from build123d import *

# Parameters (mm, degrees)
SKETCH2_R           = 3.175
SKETCH2_R_2         = 2
SKETCH2_R_3         = 1.905
SKETCH2_R_4         = 1.999999991
BOSS_EXTRUDE1_DEPTH = 5.588


with BuildPart() as part:
    # Sketch2 → Boss-Extrude1 (new body)
    with BuildSketch(Plane(origin=(0, 0, 0), x_dir=(1, 0, 0), z_dir=(0, 1, 0))):
        with BuildLine():
            Line((15.15555913, -28.018449791), (13.238676936, -27.713033224))
            ThreePointArc((13.238676936, -27.713033224), (11.241051513, -26.538356195), (10.573787778, -24.319092227))
            Line((10.573787778, -24.319092227), (12.5603, 0))
            ThreePointArc((12.5603, 0), (0.601023521, 12.545911956), (-12.502780789, 1.200670076))
            Line((-12.502780789, 1.200670076), (-16.492552312, -40.345496304))
            ThreePointArc((-16.492552312, -40.345496304), (-16.505635578, -40.527391114), (-16.51, -40.709703607))
            Line((-16.51, -40.709703607), (-16.51, -221.328861788))
            ThreePointArc((-16.51, -221.328861788), (-12.970187584, -225.680718913), (-7.988667969, -223.101301399))
            Line((-7.988667969, -223.101301399), (16.979901226, -165.677523619))
            ThreePointArc((16.979901226, -165.677523619), (17.216065593, -164.934164738), (17.295902343, -164.158289667))
            Line((17.295902343, -164.158289667), (17.295902343, -30.526810701))
            ThreePointArc((17.295902343, -30.526810701), (16.688093876, -28.878103365), (15.15555913, -28.018449791))
        make_face()
        with Locations(Location((0, 0, 0), (0, 0, 270))):
            Circle(SKETCH2_R, mode=Mode.SUBTRACT)
        with Locations(Location((-11.43, -219.075, 0), (0, 0, 270))):
            Circle(SKETCH2_R_2, mode=Mode.SUBTRACT)
        with Locations(Location((-11.43, -212.725, 0), (0, 0, 270))):
            Circle(SKETCH2_R_2, mode=Mode.SUBTRACT)
        with Locations(Location((-11.43, -206.375, 0), (0, 0, 270))):
            Circle(SKETCH2_R_2, mode=Mode.SUBTRACT)
        with Locations(Location((-11.43, -200.025, 0), (0, 0, 270))):
            Circle(SKETCH2_R_2, mode=Mode.SUBTRACT)
        with Locations(Location((-10.6553, -63.5, 0), (0, 0, 270))):
            Circle(SKETCH2_R_3, mode=Mode.SUBTRACT)
        with Locations(Location((13.485902343, -38.1, 0), (0, 0, 270))):
            Circle(SKETCH2_R_4, mode=Mode.SUBTRACT)
        with Locations(Location((13.485902343, -162.410770806, 0), (0, 0, 270))):
            Circle(SKETCH2_R_2, mode=Mode.SUBTRACT)
        with BuildLine():
            Line((10.438542905, -167.981776143), (-1.917547411, -196.39883837))
            ThreePointArc((-1.917547411, -196.39883837), (-3.730878547, -197.873050616), (-5.981020282, -197.241913761))
            Line((-5.981020282, -197.241913761), (-8.145350704, -195.219576049))
            ThreePointArc((-8.145350704, -195.219576049), (-9.634602002, -193.108963545), (-10.16, -190.579830983))
            Line((-10.16, -190.579830983), (-10.16, -156.802168612))
            ThreePointArc((-10.16, -156.802168612), (-9.585607464, -155.739610257), (-8.381999597, -155.638194561))
            Line((-8.381999597, -155.638194561), (7.135902343, -162.410768606))
            ThreePointArc((7.135902343, -162.410768606), (8.0236114, -165.648961297), (10.438542905, -167.981776143))
        make_face(mode=Mode.SUBTRACT)
        with BuildLine():
            Line((10.945902343, -147.517141807), (10.945902343, -95.265809134))
            ThreePointArc((10.945902343, -95.265809134), (10.80854708, -94.441856302), (10.411336777, -93.70701706))
            Line((10.411336777, -93.70701706), (-7.433233368, -70.749423162))
            ThreePointArc((-7.433233368, -70.749423162), (-8.766818111, -71.205159681), (-10.16, -71.417734996))
            Line((-10.16, -71.417734996), (-10.16, -145.162426346))
            ThreePointArc((-10.16, -145.162426346), (-9.122791771, -148.640463666), (-6.350002016, -150.982296599))
            Line((-6.350002016, -150.982296599), (4.488151635, -155.712459117))
            ThreePointArc((4.488151635, -155.712459117), (6.348753278, -155.779975361), (7.755557144, -154.560426346))
            Line((7.755557144, -154.560426346), (10.513009397, -149.281014802))
            ThreePointArc((10.513009397, -149.281014802), (10.836096789, -148.425250314), (10.945902343, -147.517141807))
        make_face(mode=Mode.SUBTRACT)
        with BuildLine():
            Line((-4.65837794, -58.888907788), (6.271106887, -44.827785995))
            ThreePointArc((6.271106887, -44.827785995), (6.715672228, -44.466407521), (7.273824104, -44.337182032))
            Line((7.273824104, -44.337182032), (9.675902343, -44.337182032))
            ThreePointArc((9.675902343, -44.337182032), (10.573927955, -44.70915642), (10.945902343, -45.607182032))
            Line((10.945902343, -45.607182032), (10.945902343, -84.483166252))
            ThreePointArc((10.945902343, -84.483166252), (10.087878759, -85.684488621), (8.673185126, -85.26256229))
            Line((8.673185126, -85.26256229), (-4.65837794, -68.111092212))
            ThreePointArc((-4.65837794, -68.111092212), (-3.931340897, -63.5), (-4.65837794, -58.888907788))
        make_face(mode=Mode.SUBTRACT)
        with BuildLine():
            Line((-12.415233052, -37.744377163), (-9.751235062, -10.003715048))
            ThreePointArc((-9.751235062, -10.003715048), (-2.753398549, -13.695973731), (5.127655889, -12.99492382))
            Line((5.127655889, -12.99492382), (3.069264048, -38.19397392))
            ThreePointArc((3.069264048, -38.19397392), (2.259083254, -39.854914801), (0.537695935, -40.527182032))
            Line((0.537695935, -40.527182032), (-9.886864844, -40.527182032))
            ThreePointArc((-9.886864844, -40.527182032), (-11.766801594, -39.695232914), (-12.415233052, -37.744377163))
        make_face(mode=Mode.SUBTRACT)
        with BuildLine():
            Line((-0.768822282, -44.337182032), (-10.142472044, -44.337182032))
            ThreePointArc((-10.142472044, -44.337182032), (-11.938523268, -45.081130808), (-12.682472044, -46.877182032))
            Line((-12.682472044, -46.877182032), (-12.682472044, -58.093297101))
            ThreePointArc((-12.682472044, -58.093297101), (-10.75401097, -57.726602484), (-8.814141549, -58.027158116))
            Line((-8.814141549, -58.027158116), (0.233894935, -46.386578069))
            ThreePointArc((0.233894935, -46.386578069), (0.371952228, -45.049030156), (-0.768822282, -44.337182032))
        make_face(mode=Mode.SUBTRACT)
    extrude(amount=BOSS_EXTRUDE1_DEPTH)


solid = part.part
Can you work these out from the model? Positions are in its coordinate system, mm. A direction names the side the tool comes from. Coordinates: 2 decimals unless noted, no trailing zeros. Order: outer loops, then holes, each group sorted by start corner. A loop starts at its lowest first (then second) coordinate and runs counter-clockwise, first axis right, second up. Notation, with made-up numbers: (85, -4.75) - (112, -4.75) arc R12 ccw to (112, 11.25) - close; hole circle Ø8 at (62.5, -2). An arc over 180 degrees is marked (long way). Answer as a JSON object with one key per item and string values. Group by question number.
Q1. Imagine slicing it at B-B (y = 1.8). Give the number of separate pieces and of enclosed holes in the cut face, and give its area (3 significant figures).
Q2. I need wall thicknesses on line 1 (X direction, y = 4.9, z = 118.5); line 2 (Z direction, x = 13, y = 2.75); line 3 (Z direction, x = 5.5, y = 5.35). Which ranges of each line are inside material? Lowest first, please. Write a range as from..to.
Q3. We'd pull the mould along Z, two halves only. Please class faces 1 (the face through (-16.51, 3, 130)), 2 (the face through (-12.2, 2.75, 214.57)): +Z half, -Z half, draft (parallel to the pull), parting line (faces both ways), or undercut.
Q4. Imagine slicing it at A-A (z = 17.5). Please give me the cut outline in (x, y).
Q5. On a 3-axis mill with a long thin cutter (end or side, diameter ignored), from which of +Z, -Z, +X, -X, +Y, -Y can I reach the whole of each face in a straight line? I mean faces 3 (the face through (-9.15, 2.75, 148.6)), 4 (the face through (17.296, 3, 98)). Say none if no direction works.
Q6. Will these pins go through, and if not, where does the flat tip stop? P1, Ø2.5, axis at x = -11.43, z = 219.075, coming from the +Y side; P2, Ø2.5, axis at x = 8, y = 2.5, coming from the +Z side; P3, Ø3, axis at y = 2.5, z = 173, coming from the +X side; P4, Ø3, axis at x = -7, y = 3.5, coming from the +Z side.
Determined:
{
 "1": {"separate pieces": "1", "enclosed holes": "13", "area": "3,640 mm2"},
 "2": {"line 1": "x = -16.51..-10.16, 10.95..17.3", "line 2": "z = 27.67..36.16, 40.04..160.47, 164.35..174.83", "line 3": "z = -11.29..45.82, 81.18..87.39, 155.92..161.7, 179.34..192.08"},
 "3": {"face 1": "draft", "face 2": "undercut"},
 "4": {"outline": "(-14.3, 0) - (-10.47, 0) - (-10.47, 5.59) - (-14.3, 5.59) - close; (4.76, 0) - (11.13, 0) - (11.13, 5.59) - (4.76, 5.59) - close"},
 "5": {"face 3": "+Y, -Y", "face 4": "+Z, -Z, +X, +Y, -Y"},
 "6": {"P1": "passes through", "P2": "stops at z = 189.2", "P3": "stops at x = 14.45", "P4": "stops at z = 223.98"}
}
